from build123d import *

# Parameters (mm, degrees)
SKETCH1_R          = 1.4224
EXTRUDE1_DEPTH     = 3.175
CUT_SWEEP1_PITCH   = 0.635
SKETCH6_R          = 2.3241
EXTRUDE2_DEPTH     = 2.8448
CUT_EXTRUDE1_DEPTH = 1.7859375
CHAMFER1_SIZE      = 0.23241


with BuildPart() as part:
    # Sketch1 → Extrude1 (new body)
    with BuildSketch(Plane.XY):
        Circle(SKETCH1_R)
    extrude(amount=-EXTRUDE1_DEPTH)

    # Cut-Sweep1: the profile of Sketch3 profile screwed along a right-hand helix of 6 turns, 6 arcs to a turn; built about Z, then put on its axis
    cut_sweep1_z = Axis((0, 0, 0), (0, 0, 1))
    cut_sweep1_corners = [(1.4227, 0, -0.555798205), (1.009955401, 0, -0.3175), (1.009955401, 0, -0.238125), (1.4227, 0, 0.000173205)]
    with BuildLine(mode=Mode.PRIVATE) as cut_sweep1_profile:
        Line(cut_sweep1_corners[0], cut_sweep1_corners[1])
        Line(cut_sweep1_corners[1], cut_sweep1_corners[2])
        Line(cut_sweep1_corners[2], cut_sweep1_corners[3])
        Line(cut_sweep1_corners[3], cut_sweep1_corners[0])
    cut_sweep1_cap = Face(cut_sweep1_profile.wire())
    cut_sweep1_turn_angles = [0, 30, 60, 90, 120, 150, 180, 210, 240, 270, 300, 330, 360]
    cut_sweep1_turn_weights = [1, 0.8660254037844387, 1, 0.8660254037844387, 1, 0.8660254037844387, 1, 0.8660254037844387, 1, 0.8660254037844387, 1, 0.8660254037844387, 1]
    cut_sweep1_turn_rails = [Edge.make_bspline([Vector(p[0], p[1], 0).rotate(cut_sweep1_z, cut_sweep1_turn_angles[k]) / cut_sweep1_turn_weights[k] + Vector(0, 0, p[2] + CUT_SWEEP1_PITCH * cut_sweep1_turn_angles[k] / 360) for k in range(13)], [0, 0, 0, 1, 1, 2, 2, 3, 3, 4, 4, 5, 5, 6, 6, 6], 2, cut_sweep1_turn_weights) for p in cut_sweep1_corners]
    cut_sweep1_turn_sides = [Face.make_surface_from_curves(cut_sweep1_turn_rails[p[0]], cut_sweep1_turn_rails[p[1]]) for p in [(0, 1), (1, 2), (2, 3), (3, 0)]]
    cut_sweep1 = Plane(origin=(0, 0, 0), x_dir=(0, 1, 0), z_dir=(0, 0, -1)) * Solid(Shell([*[p.moved(Location((0, 0, CUT_SWEEP1_PITCH * i))) for i in range(6) for p in cut_sweep1_turn_sides], cut_sweep1_cap, cut_sweep1_cap.rotate(cut_sweep1_z, 2160).moved(Location((0, 0, CUT_SWEEP1_PITCH * 2160 / 360)))]))
    add(cut_sweep1, mode=Mode.SUBTRACT)

    # Sketch4 → Cut-Revolve1 (revolve, cut)
    with BuildSketch(Plane(origin=(0, 0, 0), x_dir=(0, 0, -1), z_dir=(1, 0, 0)), mode=Mode.PRIVATE) as cut_revolve1_sk:
        Polygon((0.466649532, 1.4224), (0, 0.755955401), (0, 1.4224), align=None)
    revolve(cut_revolve1_sk.sketch.rotate(Axis((0, 0, 0), (0, 0, -1)), 264.795368264), axis=Axis((0, 0, 0), (0, 0, -1)), mode=Mode.SUBTRACT)

    # Sketch6 → Extrude2 (add)
    with BuildSketch(Plane(origin=(0, 0, -3.175), x_dir=(-1, 0, 0), z_dir=(0, 0, -1))):
        Circle(SKETCH6_R)
    extrude(amount=EXTRUDE2_DEPTH)

    # Sketch7 → Cut-Extrude1 (cut)
    with BuildSketch(Plane(origin=(0, 0, -6.0198), x_dir=(-1, 0, 0), z_dir=(0, 0, -1))):
        Polygon((0, 1.374815329), (-1.190625, 0.687407664), (-1.190625, -0.687407664), (0, -1.374815329), (1.190625, -0.687407664), (1.190625, 0.687407664), align=None)
    extrude(amount=-CUT_EXTRUDE1_DEPTH, mode=Mode.SUBTRACT)

    # Cut-Extrude2 cone 1 section (through the dimple's axis) → Cut-Extrude2 (revolve, cut)
    with BuildSketch(Plane(origin=(0, 0, -6.0198), x_dir=(0, 1, 0), z_dir=(1, 0, 0))):
        Polygon((0, 0), (1.374815329, 0), (0, 1.374815329), align=None)
    revolve(axis=Axis((0, 0, -6.0198), (0, 0, 1)), mode=Mode.SUBTRACT)

    # Chamfer1
    chamfer1_edges = [part.edges().sort_by_distance(p)[0] for p in [
        (2.3241, 0, -3.175),
        (2.3241, 0, -6.0198),
    ]]
    chamfer(chamfer1_edges, length=CHAMFER1_SIZE)


solid = part.part
Read the model definition and answer for the solid it produces. Units are mm, in the model's axes. A direction names the side the tool comes from. Round coordinates to 2 decimals unless told otherwise and drop trailing zeros. Loops run counter-clockwise (first coordinate to the right, second up) from the corner with the lowest first, then second, coordinate; pieces in that order, holes last. Notation, with made-up numbers: (50, -38) - (104, -38) arc R12 ccw to (104, -34) - close; hole circle Ø6 at (-13.75, 61). An arc over 180 degrees is marked (long way). One line per question, with ' | ' between items. Start each with the question number.
Q1. Section B-B on z = -3.75 is taken. Give the vertices of the cut face in (x, y), plus the area to 3 significant figures.
Q2. For a pull along X with two mould halves and no side action, classify faces 4 (the flat face through (0, 0, 0)), 5 (the cylindrical face through (0.5, -2.27, -4.58)), 6 (the flat face through (-0.587, -1.036, -5.139)) as +X half, -X half, draft (parallel to the pull), parting line (faces both ways), or undercut.
Q3. Section A-A on z = -5 is taken. Give the vertices of the cut face in (x, y).
Q4. Find the intervals of material crossed by L1, parallel to X at y = 0.1, z = -4.75; L2, parallel to Z at x = -1.1, y = 0.6; L3, parallel to Z at x = 0.05, y = 0, in increasing order.
Q5. Flat-ended cylindrical pins translate along their axes: pin 1 (1.9 mm diameter, centred on x = 0, y = 0.5, fed in from -Z); pin 2 (1.5 mm diameter, centred on x = 1.5, z = -3.5, fed in from -Y); pin 3 (1.5 mm diameter, centred on x = -1, z = -3.5, fed in from +Y). Find the tip coordinate at first contact, or state that the pin passes through.
Q6. For faces 1 (the flat face through (1.191, 0, -5)), 2 (the conical face through (0.285, -0.892, -0.126)), 3 (the flat face through (1, -1, -3.175)), determine the directions among +Z, -Z, +X, -X, +Y, -Y from which every point of the face is accessible in a straight line to the end or side of a thin tool.
Established:
1) outline: circle Ø4.65 at (0, 0) | area: 17.0 mm²
2) face 4: draft | face 5: parting line | face 6: undercut
3) outline: circle Ø4.65 at (0, 0); hole (-1.19, -0.69) - (0, -1.37) - (1.19, -0.69) - (1.19, 0.69) - (0, 1.37) - (-1.19, 0.69) - close
4) L1: -2.32 to -1.19, 1.19 to 2.32 | L2: -4.23 to -2.97, -2.61 to -2.33, -1.97 to -1.7, -1.34 to -1.06, -0.7 to -0.43 | L3: -4.23 to 0
5) pin 1: z = -6.02 | pin 2: y = -2.2 | pin 3: y = 2.31
6) face 1: -Z | face 2: +Z | face 3: none
